The listing builds one solid part. Answer for the finished solid, in the listing's coordinates (mm). A direction names the side the tool comes from. Round coordinates to 2 decimals unless told otherwise and drop trailing zeros. Order: outer loops, then holes, each group sorted by start corner. A loop starts at its lowest first (then second) coordinate and runs counter-clockwise, first axis right, second up. Notation, with made-up numbers: (44.5, -26.75) - (94.5, -26.75) arc R15 cw to (94.5, -12.75) - close; hole circle Ø9 at (28.25, 67.5). An arc over 180 degrees is marked (long way). Use CSV: the item, a comma, the result in double quotes. Start each with the question number.
Item 1: For faces 4 (the cylindrical face through (-47.036, -14.811, 52.602)), 5 (the cylindrical face through (-18, -14.8, 40.2)), 6 (the cylindrical face through (-33.04, -29.55, 39.35)), 7 (the cylindrical face through (-33.04, -0.45, 39.35)), determine the directions among +Z, -Z, +X, -X, +Y, -Y from which every point of the face is accessible in a straight line to the end or side of a thin tool.
Item 2: Find section C-C, the plane y = -2.5. Give the vertices of the cut face in (x, z), plus the area to 3 significant figures.
Item 3: Find section A-A, the plane z = 42.25. Give the vertices of the cut face in (x, y).
Item 4: Determine the mould class of faces 1 (the cylindrical face through (-16, -0.7, 55)), 2 (the cylindrical face through (-48.47, -0.28, 51.94)), 3 (the cylindrical face through (-13.985, -0.451, 45.349)) for opening direction Z: +Z half, -Z half, draft (parallel to the pull), parting line (faces both ways), or undercut.
Item 5: Flat-ended cylindrical pins translate along their axes: P1, Ø2, axis at x = -37.5, y = -20, coming from the +Z side; P2, Ø12, axis at x = -23, y = -20, coming from the +Z side. Find the tip coordinate at first contact, or state that the pin passes through.
Item 6: Straight lines are drawn through the part: line 1 along X through (y, z) = (-9.75, 46.25); line 2 along Z through (x, y) = (-30, -13); line 3 along Z through (x, y) = (-47.5, -19). For each, find the intervals that lie inside material, in ascending order. Write a range as [from, to].
Item 7: Find section B-B, the plane x = -42. Give the vertices of the cut face in (y, z), plus the area to 3 significant figures.
```python
from build123d import *

# Parameters (mm, degrees)
F1_DEPTH = 30
F2_R     = 1.5


# Not quite as in the source:
# - a feature names something its author has since deleted; it is built from what else it names


with BuildPart() as f1:
    # F0 (on Front) → F1 (new body)
    with BuildSketch(Plane.XZ):
        with BuildLine():
            ThreePointArc((-50.6280393004, 55.2302640676), (-51.6886994722, 54.7909242394), (-52.1280393004, 53.7302640676))
            Line((-52.1280393004, 53.7302640676), (-52.1280393004, 36.7302640676))
            ThreePointArc((-52.1280393004, 36.7302640676), (-51.6886994722, 35.6696038959), (-50.6280393004, 35.2302640676))
            Line((-50.6280393004, 35.2302640676), (-15.0573858261, 35.2302640676))
            ThreePointArc((-15.0573858261, 35.2302640676), (-13.9967256543, 35.6696038959), (-13.5573858261, 36.7302640676))
            Line((-13.5573858261, 36.7302640676), (-13.5573858261, 53.7302640676))
            ThreePointArc((-13.5573858261, 53.7302640676), (-13.9967256543, 54.7909242394), (-15.0573858261, 55.2302640676))
            Line((-15.0573858261, 55.2302640676), (-17.5427125633, 55.2302640676))
            Line((-17.5427125633, 55.2302640676), (-17.5427125633, 41.2777487338))
            ThreePointArc((-17.5427125633, 41.2777487338), (-17.9820523915, 40.217088562), (-19.0427125633, 39.7777487338))
            Line((-19.0427125633, 39.7777487338), (-46.6427125633, 39.7777487338))
            ThreePointArc((-46.6427125633, 39.7777487338), (-47.7033727351, 40.217088562), (-48.1427125633, 41.2777487338))
            Line((-48.1427125633, 41.2777487338), (-48.1427125633, 51.408215398))
            Line((-48.1427125633, 51.408215398), (-47.7003021707, 51.6838852273))
            ThreePointArc((-47.7003021707, 51.6838852273), (-47.032442186, 52.6176852731), (-47.2204902066, 53.7502299418))
            Line((-47.2204902066, 53.7502299418), (-48.1427125633, 55.2302640676))
            Line((-48.1427125633, 55.2302640676), (-50.6280393004, 55.2302640676))
        make_face()
    extrude(amount=F1_DEPTH)

    # F2
    f2_edges = [f1.edges().sort_by_distance(p)[0] for p in [
        (-49.385376, -30, 55.230264),
        (-51.688699, -30, 54.790924),
        (-52.128039, -30, 45.230264),
        (-51.688699, -30, 35.669604),
        (-32.842713, -30, 35.230264),
        (-13.996726, -30, 35.669604),
        (-13.557386, -30, 45.230264),
        (-13.996726, -30, 54.790924),
        (-16.300049, -30, 55.230264),
        (-17.542713, -30, 48.254006),
        (-17.982052, -30, 40.217089),
        (-32.842713, -30, 39.777749),
        (-47.703373, -30, 40.217089),
        (-48.142713, -30, 46.342982),
        (-47.921507, -30, 51.54605),
        (-47.032442, -30, 52.617685),
        (-47.681601, -30, 54.490247),
        (-49.385376, 0, 55.230264),
        (-51.688699, 0, 54.790924),
        (-52.128039, 0, 45.230264),
        (-51.688699, 0, 35.669604),
        (-32.842713, 0, 35.230264),
        (-13.996726, 0, 35.669604),
        (-13.557386, 0, 45.230264),
        (-13.996726, 0, 54.790924),
        (-16.300049, 0, 55.230264),
        (-17.542713, 0, 48.254006),
        (-17.982052, 0, 40.217089),
        (-32.842713, 0, 39.777749),
        (-47.703373, 0, 40.217089),
        (-48.142713, 0, 46.342982),
        (-47.921507, 0, 51.54605),
        (-47.032442, 0, 52.617685),
        (-47.681601, 0, 54.490247),
    ]]
    fillet(f2_edges, radius=F2_R)


solid = f1.part
```
Worked out:
1,face 4,"+Y, -Y"
1,face 5,"+Z, +Y, -Y"
1,face 6,"+Z, -Y"
1,face 7,"+Z, +Y"
2,outline,"(-52.13, 36.73) arc R1.5 ccw to (-50.63, 35.23) - (-15.06, 35.23) arc R1.5 ccw to (-13.56, 36.73) - (-13.56, 53.73) arc R1.5 ccw to (-15.06, 55.23) - (-17.54, 55.23) - (-17.54, 41.28) arc R1.5 cw to (-19.04, 39.78) - (-46.64, 39.78) arc R1.5 cw to (-48.14, 41.28) - (-48.14, 51.41) - (-47.7, 51.68) arc R1.5 ccw to (-47.22, 53.75) - (-48.14, 55.23) - (-50.63, 55.23) arc R1.5 ccw to (-52.13, 53.73) - close"
2,area,"300 mm²"
3,outline,"(-52.13, -28.5) arc R1.5 ccw to (-50.63, -30) - (-49.64, -30) arc R1.5 ccw to (-48.14, -28.5) - (-48.14, -1.5) arc R1.5 ccw to (-49.64, 0) - (-50.63, 0) arc R1.5 ccw to (-52.13, -1.5) - close; (-17.54, -28.5) arc R1.5 ccw to (-16.04, -30) - (-15.06, -30) arc R1.5 ccw to (-13.56, -28.5) - (-13.56, -1.5) arc R1.5 ccw to (-15.06, 0) - (-16.04, 0) arc R1.5 ccw to (-17.54, -1.5) - close"
4,face 1,"+Z half"
4,face 2,"undercut"
4,face 3,"draft"
5,P1,"stops at z = 39.78"
5,P2,"stops at z = 55.23"
6,line 1,"x = [-52.13, -48.14], [-17.54, -13.56]"
6,line 2,"z = [35.23, 39.78]"
6,line 3,"z = [35.23, 40.05], [51.83, 54.2]"
7,outline,"(-30, 36.73) arc R1.5 ccw to (-28.5, 35.23) - (-1.5, 35.23) arc R1.5 ccw to (0, 36.73) - (0, 38.28) arc R1.5 ccw to (-1.5, 39.78) - (-28.5, 39.78) arc R1.5 ccw to (-30, 38.28) - close"
7,area,"134 mm²"
